For this review, take the finished solid that the model builds, in its own axes (mm). A direction names the side the tool comes from. Coordinates: 2 decimals unless noted, no trailing zeros.
1. To check wall thickness, follow probe 1 along Z at (x, y) = (-88, 0); probe 2 along Z at (x, y) = (-165, -6); probe 3 along Z at (x, y) = (-142.5, -66). State the ranges of each line that lie inside material, in increasing order.
2. Mouldability with a two-part tool opening along X and no side actions: class faces 3 (the face through (-77.816, -181, 110)), 4 (the face through (10, 101, 185)), 5 (the face through (-34.523, -210.197, 9.251)) as pulls with the +X half, pulls with the -X half, needs draft (parallel to the pull), parting line crosses it, or undercut.
3. Take a section at A-A, the plane y = 118.5. Count the separate pieces of the cut face and the enclosed holes in it, then the cut area to 3 significant figures.
4. Machinability: for faces 1 (the face through (0, 44.4, 216.5)), 2 (the face through (-184.685, -210.197, 9.251)), which of the approach directions +Z, -Z, +X, -X, +Y, -Y give a long, thin tool a straight path to every point of the face, cutting with its end or side? Answer none if there is none.
5. Clearance check with flat-ended pins moving along their axes: P1, Ø10, axis at x = -84.5, y = -109.5, coming from the +Z side; P2, Ø5, axis at x = -166.5, y = 67.5, coming from the -Z side; P3, Ø10, axis at x = -173, y = 81, coming from the -Z side. State where each tip first meets the part, or that it passes through.
```python
from build123d import *

# Parameters (mm, degrees)
REVOLVE_THIN1_OUTLINE_W   = 10
REVOLVE_THIN1_OUTLINE_H   = 10
REVOLVE_THIN1_OUTLINE_W_2 = 15.028522582
REVOLVE_THIN1_OUTLINE_W_3 = 1.714910115
REVOLVE_THIN1_OUTLINE_W_4 = 33.256567303
REVOLVE_THIN1_OUTLINE_W_5 = 6.885617046
FILLET1_R                 = 30


# Read off the part's stored shape, not the designer's step: Revolve-Thin1
with BuildPart() as part:
    # Revolve-Thin1 outline → Revolve-Thin1 (revolve)
    with BuildSketch(Plane.YX):
        with Locations((215.4, 5)):
            Rectangle(REVOLVE_THIN1_OUTLINE_W, REVOLVE_THIN1_OUTLINE_H)
        with Locations((227.914261291, 5)):
            Rectangle(REVOLVE_THIN1_OUTLINE_W_2, REVOLVE_THIN1_OUTLINE_H)
        Polygon((220.4, 0), (210.4, 0), (210.4, -77.81562954), (220.4, -77.81562954), (220.4, -67.81562954), align=None)
        with Locations((240.428522582, 5)):
            Rectangle(REVOLVE_THIN1_OUTLINE_W, REVOLVE_THIN1_OUTLINE_H)
        with Locations((246.28597764, 5)):
            Rectangle(REVOLVE_THIN1_OUTLINE_W_3, REVOLVE_THIN1_OUTLINE_H)
        with Locations((227.914261291, -72.81562954)):
            Rectangle(REVOLVE_THIN1_OUTLINE_W_2, REVOLVE_THIN1_OUTLINE_H)
        Polygon((220.4, -158.368911943), (210.4, -158.651375691), (210.4, -200), (220.4, -200), (220.4, -168.372900436), align=None)
        with Locations((252.143432697, 5)):
            Rectangle(REVOLVE_THIN1_OUTLINE_W, REVOLVE_THIN1_OUTLINE_H)
        Polygon((245.428522582, -8.479983428), (235.428522582, -8.479983428), (235.428522582, -67.81562954), (235.428522582, -77.81562954), (245.428522582, -77.81562954), (245.428522582, -18.479983428), align=None)
        Polygon((235.428522582, -157.944410663), (220.4, -158.368911943), (220.4, -168.372900436), (235.428522582, -167.948399156), align=None)
        with Locations((215.4, -205)):
            Rectangle(REVOLVE_THIN1_OUTLINE_W, REVOLVE_THIN1_OUTLINE_H)
        with Locations((273.771716349, 5)):
            Rectangle(REVOLVE_THIN1_OUTLINE_W_4, REVOLVE_THIN1_OUTLINE_H)
        with Locations((246.28597764, -13.479983428)):
            Rectangle(REVOLVE_THIN1_OUTLINE_W_3, REVOLVE_THIN1_OUTLINE_H)
        Polygon((245.428522582, -157.661946915), (235.428522582, -157.944410663), (235.428522582, -167.948399156), (235.428522582, -185.030701799), (245.428522582, -185.030701799), (245.428522582, -175.030701799), align=None)
        with Locations((227.914261291, -205)):
            Rectangle(REVOLVE_THIN1_OUTLINE_W_2, REVOLVE_THIN1_OUTLINE_H)
        with Locations((293.842808523, 5)):
            Rectangle(REVOLVE_THIN1_OUTLINE_W_5, REVOLVE_THIN1_OUTLINE_H)
        Polygon((257.143432697, -8.479983428), (247.143432697, -8.479983428), (247.143432697, -18.479983428), (247.143432697, -175.030701799), (247.143432697, -185.030701799), (257.143432697, -185.030701799), align=None)
        with Locations((240.428522582, -205)):
            Rectangle(REVOLVE_THIN1_OUTLINE_W, REVOLVE_THIN1_OUTLINE_H)
        with BuildLine():
            add(Edge.make_bspline(
                [(297.285617046, 10), (298.128725715, 7.792160668), (298.973172441, 5.584730456), (300.24314277, 2.252902336), (300.665122715, 1.127420929), (301.080759322, 0)],
                knots=[0, 0, 0, 0, 0.03125, 0.03125, 0.047149929, 0.047149929, 0.047149929, 0.047149929], degree=3))
            Line((297.285617046, 10), (297.285617046, 0))
            Line((297.285617046, 0), (301.080759322, 0))
        make_face()
        with BuildLine():
            Line((297.285617046, 0), (290.4, 0))
            add(Edge.make_bspline(
                [(290.4, 0), (294.226174379, -10.019560473), (297.285617046, -20.039120946)],
                knots=[0, 0, 0, 0.100195605, 0.100195605, 0.100195605], degree=2))
            Line((297.285617046, -20.039120946), (297.285617046, 0))
        make_face()
        with Locations((246.28597764, -180.030701799)):
            Rectangle(REVOLVE_THIN1_OUTLINE_W_3, REVOLVE_THIN1_OUTLINE_H)
        with Locations((246.28597764, -205)):
            Rectangle(REVOLVE_THIN1_OUTLINE_W_3, REVOLVE_THIN1_OUTLINE_H)
        with BuildLine():
            add(Edge.make_bspline(
                [(301.080759322, 0), (301.482022229, -1.088432041), (301.877372946, -2.178671776), (303.852177937, -7.717233747), (305.338663789, -12.193981744), (308.105692918, -21.210446155), (309.386238407, -25.750161893), (311.146108373, -32.608946585), (311.705902157, -34.903411472), (312.770687134, -39.509097532), (313.275989251, -41.821845227), (317.565497999, -62.682918974), (319.49229443, -81.296552716), (319.493523861, -99.988077296), (319.493524058, -99.994036727), (319.493524058, -99.999996165)],
                knots=[0.047149929, 0.047149929, 0.047149929, 0.047149929, 0.0625, 0.0625, 0.125, 0.125, 0.1875, 0.1875, 0.21875, 0.21875, 0.25, 0.25, 0.5, 0.5, 0.500079733, 0.500079733, 0.500079733, 0.500079733], degree=3))
            Line((301.080759322, 0), (297.285617046, 0))
            Line((297.285617046, 0), (297.285617046, -20.039120946))
            add(Edge.make_bspline(
                [(297.285617046, -20.039120946), (321.701431069, -100), (297.285617046, -179.960879054)],
                knots=[0.100195605, 0.100195605, 0.100195605, 0.899804395, 0.899804395, 0.899804395], degree=2))
            Line((297.285617046, -179.960879054), (297.285617046, -200))
            Line((297.285617046, -200), (301.080759262, -200))
            add(Edge.make_bspline(
                [(319.493524058, -99.999996165), (319.493524261, -109.336842253), (319.012595, -118.691653921), (317.802753291, -130.409396195), (317.530192964, -132.755279331), (316.92393783, -137.449329338), (316.590581813, -139.794326035), (315.504714447, -146.798638914), (314.665186614, -151.437115247), (311.812847999, -165.262865698), (309.466535158, -174.360529261), (305.327261679, -187.840485904), (303.844137072, -192.30603058), (301.87370296, -197.831445048), (301.48019677, -198.916519384), (301.080759262, -200)],
                knots=[0.500079733, 0.500079733, 0.500079733, 0.500079733, 0.625, 0.625, 0.65625, 0.65625, 0.6875, 0.6875, 0.75, 0.75, 0.875, 0.875, 0.9375, 0.9375, 0.952801123, 0.952801123, 0.952801123, 0.952801123], degree=3))
        make_face()
        with Locations((273.771716349, -205)):
            Rectangle(REVOLVE_THIN1_OUTLINE_W_4, REVOLVE_THIN1_OUTLINE_H)
        with Locations((293.842808523, -205)):
            Rectangle(REVOLVE_THIN1_OUTLINE_W_5, REVOLVE_THIN1_OUTLINE_H)
        with BuildLine():
            add(Edge.make_bspline(
                [(297.285617046, -179.960879054), (294.226174379, -189.980439527), (290.4, -200)],
                knots=[0.899804395, 0.899804395, 0.899804395, 1, 1, 1], degree=2))
            Line((290.4, -200), (297.285617046, -200))
            Line((297.285617046, -200), (297.285617046, -179.960879054))
        make_face()
        with Locations((252.143432697, -205)):
            Rectangle(REVOLVE_THIN1_OUTLINE_W, REVOLVE_THIN1_OUTLINE_H)
        with BuildLine():
            Line((301.080759262, -200), (297.285617046, -200))
            Line((297.285617046, -200), (297.285617046, -210))
            add(Edge.make_bspline(
                [(301.080759262, -200), (300.664412042, -201.129348479), (300.241620682, -202.256965445), (298.971515607, -205.588939805), (298.127911115, -207.79429385), (297.285617046, -210)],
                knots=[0.952801123, 0.952801123, 0.952801123, 0.952801123, 0.96875, 0.96875, 1, 1, 1, 1], degree=3))
        make_face()
    revolve(axis=Axis((0, 0, 0), (1, 0, 0)))

    # Fillet1
    fillet1_edges = [part.edges().sort_by_distance(p)[0] for p in [
        (-210, -297.285617046, 0),
        (10, -297.285617046, 0),
    ]]
    fillet(fillet1_edges, radius=FILLET1_R)


solid = part.part
```
Results list:
1. probe 1: z = -319.23 to -309.22, -257.14 to -247.14, 247.14 to 257.14, 309.22 to 319.23
1. probe 2: z = -311.66 to -301.37, -257.07 to -247.07, -245.36 to -210.31, 210.31 to 245.36, 247.07 to 257.07, 301.37 to 311.66
1. probe 3: z = -309.21 to -298.84, -248.53 to -238.17, 238.17 to 248.53, 298.84 to 309.21
2. face 3: undercut
2. face 4: pulls with the +X half
2. face 5: needs draft
3. separate pieces: 2
3. enclosed holes: 2
3. area: 18,000 mm2
4. face 1: none
4. face 2: +X, -X
5. P1: stops at z = 301.48
5. P2: stops at z = -304.78
5. P3: stops at z = -300.8
